Verification items for the finished model (mm, model axes). A direction names the side the tool comes from. Give positions to 0.01 mm unless a question says otherwise; leave off trailing zeros. Order: outer loops, then holes, each group sorted by start corner. A loop starts at its lowest first (then second) coordinate and runs counter-clockwise, first axis right, second up. Notation, with made-up numbers: (12, 62.5) - (46, 62.5) arc R28 ccw to (46, 89.5) - close; hole circle Ø8 at (27, 18.5). An arc over 180 degrees is marked (long way). Answer as a JSON object with one key per item and string values.
```python
from build123d import *

# Parameters (mm, degrees)
SKETCH1_R           = 11.25
BOSS_EXTRUDE1_DEPTH = 5
BOSS_EXTRUDE1_DRAFT = -5
SKETCH4_R           = 11.312556682
BOSS_EXTRUDE2_DEPTH = 10
BOSS_EXTRUDE2_TAPER = 9
SKETCH3_R           = 11.25
SKETCH1_38_R        = 10
SKETCH3_7_R         = 12.25
BOSS_EXTRUDE4_DEPTH = 0.5


with BuildPart() as part:
    # Sketch1 → Boss-Extrude1 (with draft: the straight prism first)
    with BuildSketch(Plane.XY):
        Circle(SKETCH1_R)
    extrude(amount=-BOSS_EXTRUDE1_DEPTH)
    # Boss-Extrude1: the draft: its side faces are tilted about the plane it starts from
    boss_extrude1_sides = [part.faces().sort_by_distance(p)[0] for p in [
        (-11.25, 0, -2.5),
    ]]
    draft(boss_extrude1_sides, Plane.XY, BOSS_EXTRUDE1_DRAFT)

    # Sketch4 → Boss-Extrude2 (add)
    with BuildSketch(Plane(origin=(0, 0, -5), x_dir=(-1, 0, 0), z_dir=(0, 0, -1))):
        Circle(SKETCH4_R)
    extrude(amount=BOSS_EXTRUDE2_DEPTH, taper=BOSS_EXTRUDE2_TAPER)

    # Sketch3 → Loft2 section 0
    with BuildSketch(Plane(origin=(0, -2.247482777, 5.854892806), x_dir=(1, 0, 0), z_dir=(0, -0.358367949545301, 0.9335804264972015))):
        with Locations((0, 2.407379925)):
            Circle(SKETCH3_R)
    # Sketch1<38> → Loft2 section 1
    with BuildSketch(Plane.XY):
        Circle(SKETCH1_38_R)
    loft()

    # Sketch3<7> → Boss-Extrude4 (add)
    with BuildSketch(Plane(origin=(0, -2.247482777, 5.854892806), x_dir=(1, 0, 0), z_dir=(0, -0.358367949545301, 0.9335804264972015))):
        with Locations(Location((0, 2.407379925, 0), (0, 0, 270))):
            Circle(SKETCH3_7_R)
    extrude(amount=-BOSS_EXTRUDE4_DEPTH)


solid = part.part
```
(1) Gauge pin test, flat ends, axial feed: pin 1 Ø3 at (x, z) = (-10, 5.5) entering from -Y; pin 2 Ø7 at (x, y) = (5.5, -1) entering from +Z; pin 3 Ø4 at (y, z) = (-1, 3) entering from +X. Record the tip position at first contact, or that the pin passes through.
Computed values:
{"pin 1": "stops at y = -7", "pin 2": "stops at z = 7.68", "pin 3": "stops at x = 10.94"}
(2) Section check B-B (z = -9). Record the cut outline in (x, y).
Computed values:
{"outline": "circle Ø21.36 at (0, 0)"}
(3) Release check for a two-part mould opening along Z. For faces 1 (the conical face through (1.345, 10.246, -11.181)), 2 (the flat face through (-8, -7, 0)), 3 (the flat face through (0.17, 0.16, 6.78)), 4 (the conical face through (-1.424, 10.844, -3.576)) record: pulls with the +Z half, pulls with the -Z half, needs draft (parallel to the pull), parting line crosses it, or undercut.
Computed values:
{"face 1": "pulls with the -Z half", "face 2": "undercut", "face 3": "pulls with the +Z half", "face 4": "undercut"}
(4) Section check A-A (z = -1.75). Record the cut outline in (x, y), then the cut area to 3 significant figures.
Computed values:
{"outline": "circle Ø22.19 at (0, 0)", "area": "387 mm²"}
(5) Material ranges on line 1 along X through (y, z) = (-5.25, 2); line 2 along Y through (x, z) = (8.75, -7.25); line 3 along X through (y, z) = (-3.25, -8), recorded low to high. Write a range as [from, to].
Computed values:
{"line 1": "x = [-9.04, 9.04]", "line 2": "y = [-6.59, 6.59]", "line 3": "x = [-10.34, 10.34]"}
(6) Access from +Z, -Z, +X, -X, +Y, -Y to the whole of each face (thin tool, end or side, straight path). Record for faces 5 (the flat face through (0, 0, -15)), 6 (the flat face through (-1, -11, -5)).
Computed values:
{"face 5": "-Z, +X, -X, +Y, -Y", "face 6": "none"}
